```python
from build123d import *

# Parameters (mm, degrees)
F1_DEPTH = 30


with BuildPart() as f1:
    # F0 (on Top) → F1 (new body)
    with BuildSketch(Plane.XY):
        with BuildLine():
            Line((0, -47.071106), (0, 37.928894))
            ThreePointArc((0, 37.928894), (-0.732233, 39.696661), (-2.5, 40.428894))
            Line((-2.5, 40.428894), (-35, 40.428894))
            Line((-35, 40.428894), (-35, 37.928894))
            ThreePointArc((-35, 37.928894), (-34.267767, 36.161127), (-32.5, 35.428894))
            Line((-32.5, 35.428894), (-7.5, 35.428894))
            ThreePointArc((-7.5, 35.428894), (-5.732233, 34.696661), (-5, 32.928894))
            Line((-5, 32.928894), (-5, -42.071106))
            ThreePointArc((-5, -42.071106), (-5.732233, -43.838873), (-7.5, -44.571106))
            Line((-7.5, -44.571106), (-32.5, -44.571106))
            ThreePointArc((-32.5, -44.571106), (-34.267767, -45.303339), (-35, -47.071106))
            Line((-35, -47.071106), (-35, -49.571106))
            Line((-35, -49.571106), (-2.5, -49.571106))
            ThreePointArc((-2.5, -49.571106), (-0.732233, -48.838873), (0, -47.071106))
        make_face()
    extrude(amount=F1_DEPTH)


solid = f1.part
```
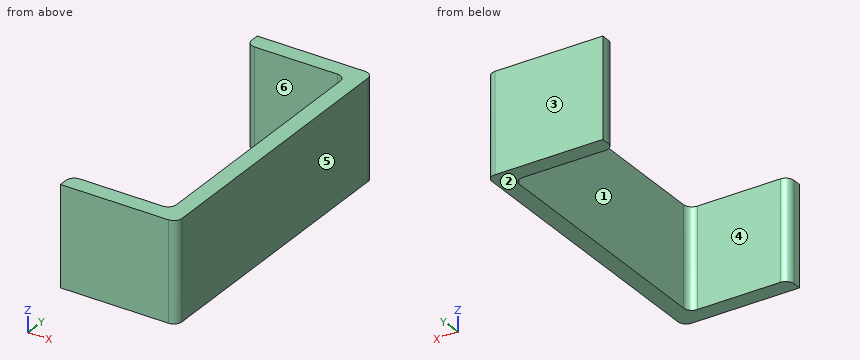
Could you check a few things on this model? Use its own coordinates, in mm. Face numbers are marked on the shaded views. A direction names the side the tool comes from. Round coordinates to 2 decimals unless told otherwise and drop trailing zeros. Loops run counter-clockwise (first coordinate to the right, second up) from the corner with the lowest first, then second, coordinate; pieces in that order, holes last. Notation, with made-up numbers: (2, -10) - (21, -10) arc R17 cw to (21, -1) - close; hole circle Ø9 at (-34, -8.5). An arc over 180 degrees is marked (long way). Use CSV: the item, a comma, the result in double quotes.
Item 1: If we section it at B-B on z = 7.5: List the corners of the cut face in (x, y) for me, then the cut area to 3 significant figures.
Here are the results:
outline,"(-35, -49.57) - (-2.5, -49.57) arc R2.5 ccw to (0, -47.07) - (0, 37.93) arc R2.5 ccw to (-2.5, 40.43) - (-35, 40.43) - (-35, 37.93) arc R2.5 ccw to (-32.5, 35.43) - (-7.5, 35.43) arc R2.5 cw to (-5, 32.93) - (-5, -42.07) arc R2.5 cw to (-7.5, -44.57) - (-32.5, -44.57) arc R2.5 ccw to (-35, -47.07) - close"
area,"747 mm²"
Item 2: If we section it at C-C on y = 5: List the corners of the cut face in (x, z) for me.
Here are the results:
outline,"(-5, 0) - (0, 0) - (0, 30) - (-5, 30) - close"
Item 3: If we mould it in two halves opening along Y, with no side actions, what happens to the marked faces 1, 2, 3 and 4? For each: pulls with the +Y half, pulls with the -Y half, needs draft (parallel to the pull), parting line crosses it, or undercut.
Here are the results:
face 1,"undercut"
face 2,"needs draft"
face 3,"pulls with the +Y half"
face 4,"undercut"
Item 4: Will these pins go through, and if not, where does the flat tip stop? pin 1 (5 mm diameter, centred on y = 15, z = 4, fed in from -X); pin 2 (10 mm diameter, centred on x = -8, y = -17, fed in from +Z).
Here are the results:
pin 1,"stops at x = -5"
pin 2,"stops at z = 30"
Item 5: If we section it at A-A on x = -29: List the corners of the cut face in (y, z) for me.
Here are the results:
outline,"(-49.57, 0) - (-44.57, 0) - (-44.57, 30) - (-49.57, 30) - close; (35.43, 0) - (40.43, 0) - (40.43, 30) - (35.43, 30) - close"
Item 6: I need wall thicknesses on L1, parallel to Y at x = -32, z = 16.75; L2, parallel to X at y = 16.5, z = 22.25; L3, parallel to Y at x = -7, z = 16.75. Which ranges of each line are inside material? Lowest first, please. Write a range as [from, to].
Here are the results:
L1,"y = [-49.57, -44.57], [35.43, 40.43]"
L2,"x = [-5, 0]"
L3,"y = [-49.57, -44.52], [35.38, 40.43]"
Item 7: For the marked faces 5 and 6, which set-ups out of +Z, -Z, +X, -X, +Y, -Y let a thin tool reach every point of the face, with its end or its side?
Here are the results:
face 5,"+Z, -Z, +X, +Y, -Y"
face 6,"+Z, -Z, -X"
